Study the drawing (mm; zero at the part's minimum x, y, z) and answer. Round coordinates to 2 decimals unless told otherwise and drop trailing zeros. Order: outer loops, then holes, each group sorted by start corner. A loop starts at its lowest first (then second) coordinate and runs counter-clockwise, first axis right, second up. Notation, with made-up numbers: (16, 19.5) - (64, 19.5) arc R27 cw to (64, 35.5) - close; hole circle Ø11 at (2, 22). An arc over 180 degrees is marked (long way). Use one line per item in the form item = value. Start each with the question number.
Q1. Given P1, Ø3, axis at x = 11.5, y = 12, coming from the -Z side, flat-ended and moving along its own axis, determine where the tip first touches the part or whether it passes through.
Q2. For a pull along X with two mould halves and no side action, classify the marked faces 1, 2 and 3 as +X half, -X half, draft (parallel to the pull), parting line (faces both ways), or undercut.
Q3. Find the intervals of material crossed by line 1 (Y direction, x = 10, z = 2); line 2 (Z direction, x = 9, y = 14); line 3 (Y direction, x = 12, z = 6.5), in increasing order. Write a range as [from, to].
Q4. The part is cut by section A-A on y = 10. Determine the outline of the cut face in (x, z), plus the area to 3 significant figures.
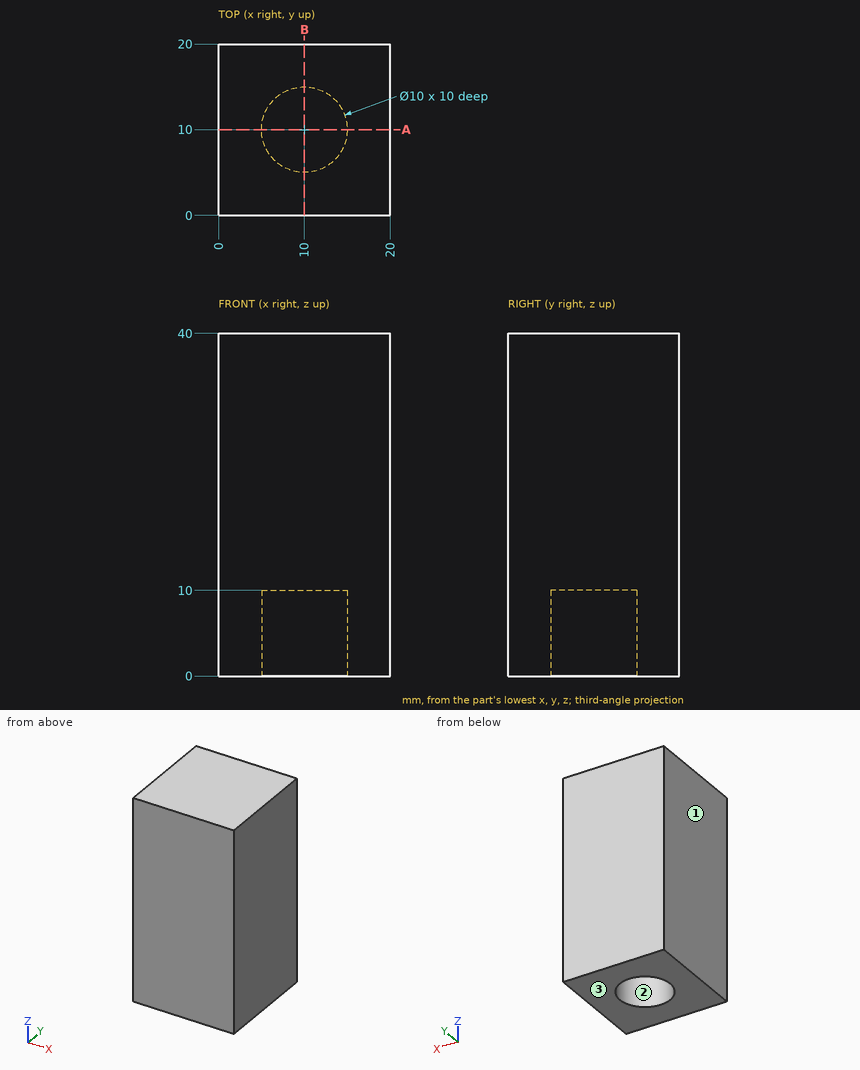
Found:
q1.P1 = 10
q2.face_1 = -X half
q2.face_2 = undercut
q2.face_3 = draft
q3.line_1 = [0, 5], [15, 20]
q3.line_2 = [10, 40]
q3.line_3 = [0, 5.42], [14.58, 20]
q4.outline = (0, 0) - (5, 0) - (5, 10) - (15, 10) - (15, 0) - (20, 0) - (20, 40) - (0, 40) - close
q4.area = 700 mm²
